Check sheet for the modelled part. Datum: model origin and axes. Units: mm. A direction names the side the tool comes from. Round coordinates to 2 decimals unless told otherwise and drop trailing zeros. Loops run counter-clockwise (first coordinate to the right, second up) from the corner with the lowest first, then second, coordinate; pieces in that order, holes last. Notation, with made-up numbers: M 24,37.5 L 71,37.5 A11 ccw 71,50.5 Z; hole C -1,39.5 d6. An arc over 180 degrees is marked long. One line per question, with ' | ' between items. Start each with the question number.
(1) Section check B-B (x = 1.5). Record the boundary of the cut face in (y, z), and give its area (3 significant figures).
(2) Section check C-C (y = 11.5). Record the boundary of the cut face in (x, z), and give its area (3 significant figures).
(3) Section check A-A (z = 9.25). Record the boundary of the cut face in (x, y).
(4) Tool access check on faces 1 (the face through (5, -19, 4.3)), 2 (the face through (5, -23, 7.3)), 3 (the face through (5, 23, 7.3)). Record the directions out of +Z, -Z, +X, -X, +Y, -Y that give a thin tool (end or side, any length) a straight path to the whole face; none if there is none.
(5) Section check D-D (z = 11.75). Record the boundary of the cut face in (x, y).
(6) Go/stop test with flat-tipped pins: P1, Ø2, axis at x = 5.5, y = -2.5, coming from the +Z side; P2, Ø1, axis at x = 6.5, y = -18, coming from the +Z side; P3, Ø2, axis at y = 15.5, z = 10, coming from the +X side. Record where each tip stops, or that it passes through.
(7) Thickness scan on probe 1 along Z at (x, y) = (9, 26.5); probe 2 along Y at (x, z) = (1.25, 5.75); probe 3 along Y at (x, z) = (2.5, 5.25). Record the ranges inside material, lowest first. Write a range as [from, to].
```python
from build123d import *

# Parameters (mm, degrees)
EXTRUDE_1_DEPTH = 10
FILLET_1_R      = 10


with BuildPart() as part:
    # 草图1 → 凸台-拉伸1 (new body)
    with BuildSketch(Plane(origin=(0, 0, 0), x_dir=(0, 0, -1), z_dir=(1, 0, 0))):
        with BuildLine():
            Line((-4.3, 9.028288874), (-4.3, 29.028288874))
            Line((-4.3, 29.028288874), (-7.3, 29.028288874))
            Line((-7.3, 29.028288874), (-7.3, 12.028288874))
            ThreePointArc((-7.3, 12.028288874), (-12.261361814, 6.901357817), (-14.070171756, 0))
            Line((-14.070171756, 0), (-10, 0))
            ThreePointArc((-10, 0), (-8.455767263, 5.338539126), (-4.3, 9.028288874))
        make_face()
    extrude_1 = extrude(amount=EXTRUDE_1_DEPTH)

    # 镜向1: 凸台-拉伸1 across plane
    add(extrude_1.mirror(Plane(origin=(10, 0, 14.070171756), x_dir=(0, 0, 1), z_dir=(0, 1, 0))))

    # 圆角1
    fillet_1_edges = [part.edges().sort_by_distance(p)[0] for p in [
        (5, 12.028288874, 7.3),
        (5, -12.028288874, 7.3),
    ]]
    fillet(fillet_1_edges, radius=FILLET_1_R)


solid = part.part
```
The answers:
1) outline: M -29.03,4.3 L -9.03,4.3 A10 cw 9.03,4.3 L 29.03,4.3 L 29.03,7.3 L 16.74,7.3 A10 cw 9.78,10.11 A14.07 ccw -9.78,10.11 A10 cw -16.74,7.3 L -29.03,7.3 Z | area: 221 mm²
2) outline: M 0,4.3 L 10,4.3 L 10,8.78 L 0,8.78 Z | area: 44.8 mm²
3) outline: M 0,-10.8 L 10,-10.8 L 10,-3.8 L 0,-3.8 Z; M 0,3.8 L 10,3.8 L 10,10.8 L 0,10.8 Z
4) face 1: -Z, +X, -X, +Y, -Y | face 2: +Z, +X, -X, -Y | face 3: +Z, +X, -X, +Y
5) outline: M 0,-7.74 L 10,-7.74 L 10,7.74 L 0,7.74 Z
6) P1: z = 13.99 | P2: z = 7.3 | P3: through
7) probe 1: [4.3, 7.3] | probe 2: [-29.03, -8.18], [8.18, 29.03] | probe 3: [-29.03, -8.51], [8.51, 29.03]
